Source: CAD feature listing. Evaluate the final solid. Frame: model axes, mm. A direction names the side the tool comes from. Round coordinates to 2 decimals unless told otherwise and drop trailing zeros. Order: outer loops, then holes, each group sorted by start corner. A loop starts at its lowest first (then second) coordinate and runs counter-clockwise, first axis right, second up. Notation, with made-up numbers: (-30.75, -30) - (-26.75, -30) arc R10 ccw to (-26.75, -11) - close; hole circle Ø9 at (33, -16.5). An arc over 180 degrees is marked (long way). Return JSON: item names as keys, results as strings. Group by question number.
1) Access query for faces 1 (the flat face through (-44.2, -1, 45)), 2 (the flat face through (-45, 0, 44)). Directions: +Z, -Z, +X, -X, +Y, -Y. A direction counts if a zero-diameter tool reaches every point of the face in a straight line with its end or side. Return the directions, or none.
2) Section C-C, the plane x = 20. Return loops of the section in (y, z).
3) Ray query, line 1 (X direction, y = 0.5, z = 71.5); line 2 (Z direction, x = -23, y = -12); line 3 (Y direction, x = -28, z = 7.5). Return the intervals inside material, ascending. Write a range as from..to.
4) Contact query for flat-ended pins moving along their axis: P1, Ø10, axis at x = 21, y = -32, coming from the +Z side; P2, Ø6, axis at x = -12.5, z = 35.5, coming from the -Y side; P3, Ø1.5, axis at y = 22.5, z = 14, coming from the +X side. Output: stop coordinate, or through.
5) Section B-B, the plane y = 37.5. Return loops of the section in (x, z).
```python
from build123d import *

# Parameters (mm, degrees)
F0_W     = 89.2000017881
F0_H     = 89.2
F1_DEPTH = 0.8
F2_DEPTH = 90


# Not quite as in the source:
# - ends of sketch curves that miss each other by under 0.0002 mm in the source are joined


with BuildPart() as f1:
    # F0 (on Top) → F1 (new body)
    with BuildSketch(Plane.XY):
        with Locations((0.3999991059, -0.4)):
            Rectangle(F0_W, F0_H)
    extrude(amount=F1_DEPTH)

    # F0 (on Top) → F2 (join)
    with BuildSketch(Plane.XY):
        Polygon((-45, -45), (-44.2000017881, -45), (-44.2000017881, 44.2), (-45.0000017881, 44.2), align=None)
        Polygon((-44.2000017881, 44.2), (44.9999982119, 44.2), (45, 45), (-45, 45), (-45, 44.2), align=None)
    extrude(amount=F2_DEPTH)


solid = f1.part
```
Geometry check:
{
 "1": {"face 1": "+Z, +X, -Y", "face 2": "+Z, -Z, -X, +Y, -Y"},
 "2": {"outline": "(-45, 0) - (45, 0) - (45, 90) - (44.2, 90) - (44.2, 0.8) - (-45, 0.8) - close"},
 "3": {"line 1": "-45..-44.2", "line 2": "0..0.8", "line 3": "44.2..45"},
 "4": {"P1": "z = 0.8", "P2": "y = 44.2", "P3": "x = -44.2"},
 "5": {"outline": "(-45, 0) - (45, 0) - (45, 0.8) - (-44.2, 0.8) - (-44.2, 90) - (-45, 90) - close"}
}
